Part model, mm, in its own coordinate system. A direction names the side the tool comes from. Give positions to 0.01 mm unless a question says otherwise; leave off trailing zeros. Order: outer loops, then holes, each group sorted by start corner. A loop starts at its lowest first (then second) coordinate and runs counter-clockwise, first axis right, second up. Notation, with made-up numbers: (11.5, -32) - (62.5, -32) arc R21 ccw to (62.5, -25) - close; hole circle Ø7 at (-31.5, 55). An arc over 180 degrees is marked (long way). Use one line per item in the form item = value. Start each with the question number.
1. Band-saw the part on B-B, the plane x = -1.5. List the corners of the cut face in (y, z).
2. Pull direction Z, two halves, no side cores. Call faces 1 (the face through (-12.771, -0.607, -1.926)), 2 (the face through (-17.78, 2, 2)), 3 (the face through (0.25, -6.2, 1.38)): +Z half, -Z half, draft (parallel to the pull), parting line (faces both ways), or undercut.
3. Drill centre lines: line 1 (Y direction, x = 10.25, z = 0); line 2 (Z direction, x = 12, y = -0.5); line 3 (Z direction, x = -9.5, y = -5.25). Where is each one in solid material? Low to high.
4. Pin check, flat tips, straight feed: P1, Ø2.5, axis at y = 0, z = 0, coming from the +X side; P2, Ø5, axis at x = -7, y = -4, coming from the +Z side. Stop position of each tip, or through.
5. Band-saw the part on D-D, the plane z = -3.25. List the corners of the cut face in (x, y).
6. Band-saw the part on A-A, the plane x = 12. List the corners of the cut face in (y, z).
7. Tool access for faces 4 (the face through (-6.617, 0.342, 0.076)), 5 (the face through (12.771, -0.607, -1.926)): list every direction of +Z, -Z, +X, -X, +Y, -Y with a clear straight run to the whole face (end or side of a thin tool).
8. Band-saw the part on C-C, the plane y = -2.5. List the corners of the cut face in (x, z).
from build123d import *

# Parameters (mm, degrees)
SKETCH1_R           = 6.35
BOSS_EXTRUDE1_DEPTH = 17.78


with BuildPart() as part:
    # Sketch1 → Boss-Extrude1 (new, symmetric)
    with BuildSketch(Plane(origin=(0, 0, 0), x_dir=(0, 0, -1), z_dir=(1, 0, 0))):
        Circle(SKETCH1_R)
    extrude(amount=BOSS_EXTRUDE1_DEPTH, both=True)

    # Sketch4 → Tap Drill for #10-32 Tap1 (revolve, cut)
    with BuildSketch(Plane(origin=(17.78, 0, 0), x_dir=(0, 0, -1), z_dir=(0, 1, 0))):
        Polygon((0, 0), (0, 11.373317848), (2.0193, 10.16), (2.0193, 0), align=None)
    tap_drill_for_10_32_tap1 = revolve(axis=Axis((24.13, 0, 0), (-1, 0, 0)), mode=Mode.SUBTRACT)

    # Mirror1: Tap Drill for #10-32 Tap1 across plane
    add(tap_drill_for_10_32_tap1.mirror(Plane(origin=(0, 0, 0), x_dir=(0, 0, 1), z_dir=(1, 0, 0))), mode=Mode.SUBTRACT)


solid = part.part
From the geometry:
q1.outline = circle Ø12.7 at (0, 0)
q2.face_1 = undercut
q2.face_2 = draft
q2.face_3 = parting line
q3.line_1 = -6.35 to -2.02, 2.02 to 6.35
q3.line_2 = -6.33 to -1.96, 1.96 to 6.33
q3.line_3 = -3.57 to 3.57
q4.P1 = 7.16
q4.P2 = 6.17
q5.outline = (-17.78, -5.46) - (17.78, -5.46) - (17.78, 5.46) - (-17.78, 5.46) - close
q6.outline = circle Ø12.7 at (0, 0); hole circle Ø4.04 at (0, 0)
q7.face_4 = -X
q7.face_5 = +X
q8.outline = (-17.78, -5.84) - (17.78, -5.84) - (17.78, 5.84) - (-17.78, 5.84) - close
